from build123d import *

# Parameters (mm, degrees)
BOSS_EXTRUDE1_DEPTH = 6.35
BOSS_EXTRUDE2_DEPTH = 44.45
SKETCH4_W           = 12.7
SKETCH4_H           = 31.75
BOSS_EXTRUDE4_DEPTH = 50.8
SKETCH5_W           = 22.86
SKETCH5_H           = 38.1
CUT_EXTRUDE1_DEPTH  = 44.45
FILLET3_R           = 17.78


with BuildPart() as part:
    # Sketch1 → Boss-Extrude1 (new body)
    with BuildSketch(Plane(origin=(0, 0, 0), x_dir=(1, 0, 0), z_dir=(0, 1, 0))):
        with BuildLine():
            Line((-88.9, -76.2), (88.9, -76.2))
            ThreePointArc((88.9, -76.2), (114.692568029, -23.564058203), (111.741834586, 34.977312694))
            Line((111.741834586, 34.977312694), (88.9, 107.95))
            Line((88.9, 107.95), (63.5, 107.95))
            Line((63.5, 107.95), (63.5, 76.2))
            Line((63.5, 76.2), (-63.5, 76.2))
            Line((-63.5, 76.2), (-63.5, 107.95))
            Line((-63.5, 107.95), (-76.2, 107.95))
            Line((-76.2, 107.95), (-88.9, 76.2))
            ThreePointArc((-88.9, 76.2), (-117.088214608, 0), (-88.9, -76.2))
        make_face()
        with BuildLine():
            Line((-101.250873324, 25.4), (-86.010873324, 25.4))
            Line((-86.010873324, 25.4), (-86.010873324, -25.4))
            Line((-86.010873324, -25.4), (-101.250873324, -25.4))
            ThreePointArc((-101.250873324, -25.4), (-104.388214608, 0), (-101.250873324, 25.4))
        make_face(mode=Mode.SUBTRACT)
        with BuildLine():
            Line((86.010873324, -25.4), (101.250873324, -25.4))
            ThreePointArc((101.250873324, -25.4), (104.388214608, 0), (101.250873324, 25.4))
            Line((101.250873324, 25.4), (86.010873324, 25.4))
            Line((86.010873324, 25.4), (86.010873324, -25.4))
        make_face(mode=Mode.SUBTRACT)
    extrude(amount=BOSS_EXTRUDE1_DEPTH)

    # Sketch2 → Boss-Extrude2 (add)
    with BuildSketch(Plane(origin=(0, 6.35, 0), x_dir=(1, 0, 0), z_dir=(0, 1, 0))):
        with BuildLine():
            Line((-88.9, -76.2), (88.9, -76.2))
            ThreePointArc((88.9, -76.2), (114.692568029, -23.564058203), (111.741834586, 34.977312694))
            Line((111.741834586, 34.977312694), (88.9, 107.95))
            Line((88.9, 107.95), (63.5, 107.95))
            Line((63.5, 107.95), (63.5, 76.2))
            Line((63.5, 76.2), (-63.5, 76.2))
            Line((-63.5, 76.2), (-63.5, 107.95))
            Line((-63.5, 107.95), (-76.2, 107.95))
            Line((-76.2, 107.95), (-88.9, 76.2))
            ThreePointArc((-88.9, 76.2), (-117.088214608, 0), (-88.9, -76.2))
        make_face()
        with BuildLine():
            Line((-82.853179474, -63.5), (82.853179474, -63.5))
            ThreePointArc((82.853179474, -63.5), (104.388214608, 0), (82.853179474, 63.5))
            Line((82.853179474, 63.5), (-82.853179474, 63.5))
            ThreePointArc((-82.853179474, 63.5), (-104.388214608, 0), (-82.853179474, -63.5))
        make_face(mode=Mode.SUBTRACT)
    extrude(amount=BOSS_EXTRUDE2_DEPTH)

    # Sketch4 → Boss-Extrude4 (add)
    with BuildSketch(Plane(origin=(0, 50.8, 0), x_dir=(1, 0, 0), z_dir=(0, 1, 0))):
        with Locations((57.15, 92.075)):
            Rectangle(SKETCH4_W, SKETCH4_H)
    extrude(amount=-BOSS_EXTRUDE4_DEPTH)

    # Sketch5 → Cut-Extrude1 (cut)
    with BuildSketch(Plane(origin=(0, 50.8, 0), x_dir=(1, 0, 0), z_dir=(0, 1, 0))):
        with Locations((71.423179474, 82.55)):
            Rectangle(SKETCH5_W, SKETCH5_H)
    extrude(amount=-CUT_EXTRUDE1_DEPTH, mode=Mode.SUBTRACT)

    # Fillet3
    fillet3_edges = [part.edges().sort_by_distance(p)[0] for p in [
        (50.8, 25.4, -76.2),
        (-63.5, 25.4, -76.2),
    ]]
    fillet(fillet3_edges, radius=FILLET3_R)


solid = part.part
Can you work these out from the model? Positions are in its coordinate system, mm. A direction names the side the tool comes from. Give positions to 0.01 mm unless a question says otherwise; leave off trailing zeros. Loops run counter-clockwise (first coordinate to the right, second up) from the corner with the lowest first, then second, coordinate; pieces in that order, holes last. Notation, with made-up numbers: (-40, 19) - (-35, 19) arc R22 ccw to (-35, 34) - close; hole circle Ø4 at (62, 60.25). An arc over 180 degrees is marked (long way). Return JSON: item names as keys, results as strings.
1. If I drill on line 1 (Z direction, x = -27, y = 19.5); line 2 (Z direction, x = -65, y = 44); line 3 (X direction, y = 14, z = 0.5), over which ranges is the centre line in solid material (lowest first)?
Output values:
{"line 1": "z = -76.2 to -63.5, 63.5 to 76.2", "line 2": "z = -107.95 to -63.5, 63.5 to 76.2", "line 3": "x = -117.09 to -104.39, 104.39 to 117.09"}
2. We'd pull the mould along Z, two halves only. Please class faces 1 (the face through (100.48, 25.04, -70.95)), 2 (the face through (-1, 50.8, -64)), 3 (the face through (-10, 28, -63.5)), 4 (the face through (82.853, 29, -82)): +Z half, -Z half, draft (parallel to the pull), parting line (faces both ways), or undercut.
Output values:
{"face 1": "-Z half", "face 2": "draft", "face 3": "undercut", "face 4": "undercut"}
3. I want a section at C-C on x = -11.5. Please give me the cut outline in (y, z).
Output values:
{"outline": "(0, -76.2) - (50.8, -76.2) - (50.8, -63.5) - (6.35, -63.5) - (6.35, 63.5) - (50.8, 63.5) - (50.8, 76.2) - (0, 76.2) - close"}
4. For faces 5 (the face through (-58.153, 25.044, -81.27)), 6 (the face through (71, 29, -101.6)), 7 (the face through (86.011, 3, 0)), which set-ups out of +Z, -Z, +X, -X, +Y, -Y let a thin tool reach every point of the face, with its end or its side?
Output values:
{"face 5": "-Z, +Y, -Y", "face 6": "+Y", "face 7": "+Y, -Y"}
5. I want a section at D-D on z = 53.5. Please give me the cut outline in (x, y), and give its area (3 significant figures).
Output values:
{"outline": "(-104.15, 0) - (104.15, 0) - (104.15, 50.8) - (89.64, 50.8) - (89.64, 6.35) - (-89.64, 6.35) - (-89.64, 50.8) - (-104.15, 50.8) - close", "area": "2,610 mm²"}
6. I'm going to push flat-ended pins straight in: pin 1 Ø4 at (y, z) = (22.5, -98) entering from +X; pin 2 Ø10 at (x, z) = (3.5, 57.5) entering from +Y; pin 3 Ø1.5 at (y, z) = (24.5, 36) entering from -X. Where does each tip first touch, or does it pass through?
Output values:
{"pin 1": "stops at x = 92.64", "pin 2": "stops at y = 6.35", "pin 3": "stops at x = -111.66"}
7. I want a section at A-A on y = 29. Please give me the cut outline in (x, z), and give its area (3 significant figures).
Output values:
{"outline": "(-88.9, -76.2) - (-76.2, -107.95) - (-63.5, -107.95) - (-63.5, -93.98) arc R17.78 cw to (-45.72, -76.2) - (33.02, -76.2) arc R17.78 cw to (50.8, -93.98) - (50.8, -107.95) - (88.9, -107.95) - (111.74, -34.98) arc R117.09 ccw to (88.9, 76.2) - (-88.9, 76.2) arc R117.09 ccw to start; hole (-82.85, -63.5) - (59.99, -63.5) - (59.99, -101.6) - (82.85, -101.6) - (82.85, -63.5) arc R104.39 ccw to (82.85, 63.5) - (-82.85, 63.5) arc R104.39 ccw to start", "area": "9,570 mm²"}
8. I want a section at B-B on z = 7.5. Please give me the cut outline in (x, y), and give its area (3 significant figures).
Output values:
{"outline": "(-116.85, 0) - (-104.12, 0) - (-104.12, 50.8) - (-116.85, 50.8) - close; (-86.01, 0) - (86.01, 0) - (86.01, 6.35) - (-86.01, 6.35) - close; (104.12, 0) - (116.85, 0) - (116.85, 50.8) - (104.12, 50.8) - close", "area": "2,390 mm²"}
